Could you check a few things on this model? Use its own coordinates, in mm. A direction names the side the tool comes from. Give positions to 0.01 mm unless a question says otherwise; leave off trailing zeros. Order: outer loops, then holes, each group sorted by start corner. A loop starts at its lowest first (then second) coordinate and runs counter-clockwise, first axis right, second up.
(1) Will these pins go through, and if not, where does the flat tip stop? pin 1 (3 mm diameter, centred on x = 20.5, y = 649, fed in from +Z); pin 2 (15 mm diameter, centred on x = 18.5, z = 66, fed in from +Y).
(2) Imagine slicing it at B-B, the plane z = 82.5. Write out the boundary of the cut face in (x, y), then the cut area to 3 significant figures.
(3) On a 3-axis mill with a long thin cutter (end or side, diameter ignored), from which of +Z, -Z, +X, -X, +Y, -Y can I reach the whole of each face in a straight line? I mean faces 1 (the flat face through (0, 490, 28)), 2 (the flat face through (25, 515, 50.8)). Say none if no direction works.
(4) Imagine slicing it at C-C, the plane y = 283. Write out the boundary of the cut face in (x, z), then the cut area to 3 significant figures.
(5) If I drill on probe 1 along Y at (x, z) = (25, 11); probe 2 along Y at (x, z) = (25.4, 12.5) (3 decimals); probe 3 along X at (y, z) = (152, 18), over which ranges is the centre line in solid material (lowest first)?
(6) Imagine slicing it at A-A, the plane x = 37.5. Write out the boundary of the cut face in (y, z).
from build123d import *

# Parameters (mm, degrees)
F0_W     = 50.8
F0_H     = 1016
F0_R     = 3.175
F1_DEPTH = 50.8
F2_W     = 50.8
F2_H     = 50.8
F3_DEPTH = 101.6


with BuildPart() as f1:
    # F0 (on Top) → F1 (new body)
    with BuildSketch(Plane.XY):
        with Locations((25.4, 508)):
            Rectangle(F0_W, F0_H)
        with Locations((25.4, 152.4)):
            Circle(F0_R, mode=Mode.SUBTRACT)
        with Locations((25.4, 863.6)):
            Circle(F0_R, mode=Mode.SUBTRACT)
    extrude(amount=F1_DEPTH)

    # F2 (on face) → F3 (join)
    with BuildSketch(Plane(origin=(0, 0, 0), x_dir=(1, 0, 0), z_dir=(0, 0, -1))):
        with Locations((25.4, 25.4)):
            Rectangle(F2_W, F2_H)
    extrude(amount=-F3_DEPTH)


solid = f1.part
Answer block:
1. pin 1: stops at z = 50.8
1. pin 2: stops at y = 0
2. outline: (0, -50.8) - (50.8, -50.8) - (50.8, 0) - (0, 0) - close
2. area: 2,580 mm2
3. face 1: +Z, -Z, -X, +Y, -Y
3. face 2: +Z, +X, -X, +Y
4. outline: (0, 0) - (50.8, 0) - (50.8, 50.8) - (0, 50.8) - close
4. area: 2,580 mm2
5. probe 1: y = -50.8 to 149.25, 155.55 to 860.45, 866.75 to 1016
5. probe 2: y = -50.8 to 149.225, 155.575 to 860.425, 866.775 to 1016
5. probe 3: x = 0 to 22.25, 28.55 to 50.8
6. outline: (-50.8, 0) - (1016, 0) - (1016, 50.8) - (0, 50.8) - (0, 101.6) - (-50.8, 101.6) - close
